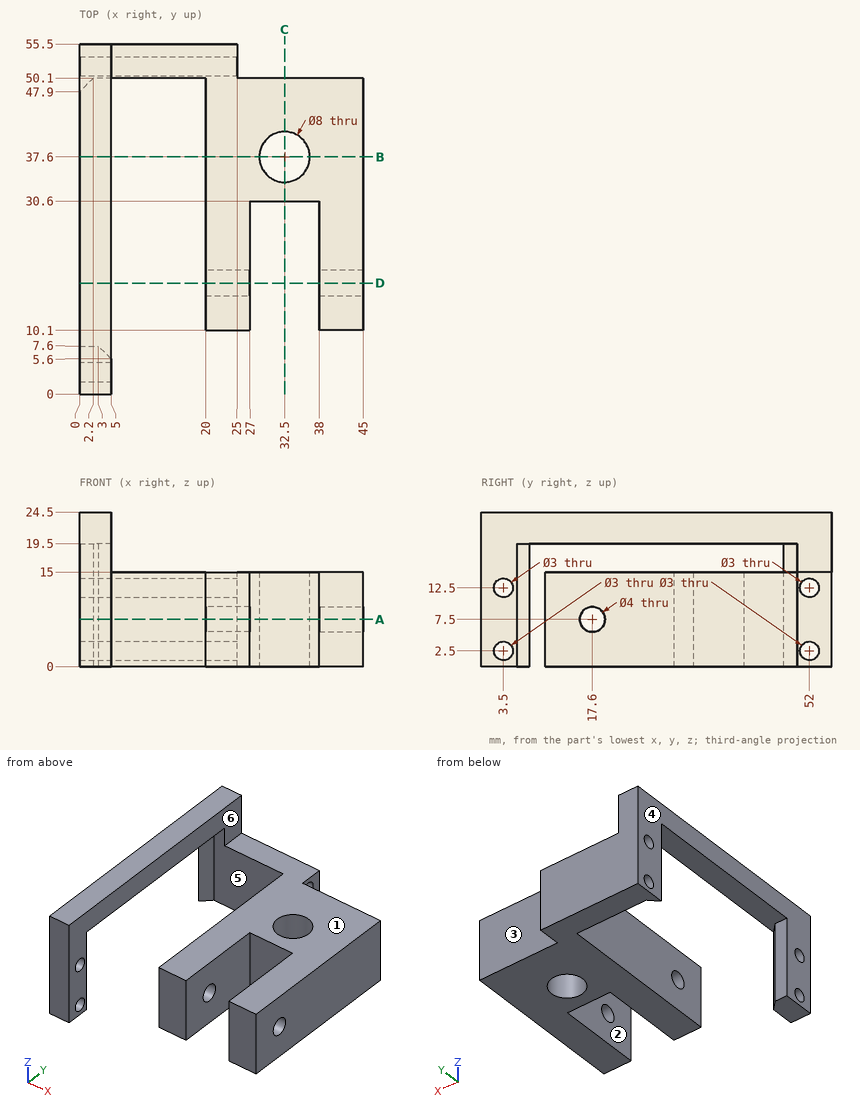
Could you check a few things on this drawing? It's one solid part, dimensions in mm from its lowest x, y, z. A direction names the side the tool comes from. Round coordinates to 2 decimals unless told otherwise and drop trailing zeros. Order: outer loops, then holes, each group sorted by start corner. A loop starts at its lowest first (then second) coordinate and runs counter-clockwise, first axis right, second up. Notation, with made-up numbers: M 32.25,88 L 74.25,88 A16 cw 74.25,113 Z; hole C -15.75,29.5 d5. An arc over 180 degrees is marked long. One line per question, with ' | ' between items. Start each with the question number.
(1) Suppose I cut it at C-C on x = 32.5. List the corners of the cut face in (y, z) for me, then the cut area to 4 significant figures.
(2) Suppose I cut it at B-B on y = 37.6. List the corners of the cut face in (x, z) for me, then the cut area to 3 significant figures.
(3) Thinking about a two-plate mould opening in X: for the marked faces 4, 5 and 6, which applies, +X half, -X half, draft (parallel to the pull), parting line (faces both ways), or undercut?
(4) Suppose I cut it at D-D on y = 17.6. List the corners of the cut face in (x, z) for me.
(5) Please list where these lines run through material, in increasing order: line 1 along Z through (x, y) = (7.25, 52); line 2 along Z through (x, y) = (38, 38.5); line 3 along Y through (x, z) = (32.5, 10.5).
(6) For P1, Ø12, axis at x = 33, z = 11, coming from the +Y side; P2, Ø2, axis at y = 39.5, z = 8.5, coming from the -X side; P3, Ø20, axis at x = 19, y = 32.5, coming from the +Z side; P4, Ø3.5, axis at y = 52, z = 2.5, coming from the -X side, each with a flat end and sliding along its axis, tell me the tip position at first contact or that it passes through.
(7) For the marked faces 1, 2 and 3, which set-ups out of +Z, -Z, +X, -X, +Y, -Y let a thin tool reach every point of the face, with its end or its side?
(8) Suppose I cut it at A-A on z = 7.5. List the corners of the cut face in (x, y) for me, then the cut area to 3 significant figures.
Geometry results:
1) outline: M 30.6,0 L 33.6,0 L 33.6,15 L 30.6,15 Z; M 41.6,0 L 50.1,0 L 50.1,15 L 41.6,15 Z | area: 172.5 mm²
2) outline: M 0,19.5 L 5,19.5 L 5,24.5 L 0,24.5 Z; M 20,0 L 28.5,0 L 28.5,15 L 20,15 Z; M 36.5,0 L 45,0 L 45,15 L 36.5,15 Z | area: 280 mm²
3) face 4: -X half | face 5: undercut | face 6: +X half
4) outline: M 0,19.5 L 5,19.5 L 5,24.5 L 0,24.5 Z; M 20,0 L 27,0 L 27,5.5 L 20,5.5 Z; M 20,9.5 L 27,9.5 L 27,15 L 20,15 Z; M 38,0 L 45,0 L 45,5.5 L 38,5.5 Z; M 38,9.5 L 45,9.5 L 45,15 L 38,15 Z
5) line 1: 0 to 1, 4 to 11, 14 to 15 | line 2: 0 to 15 | line 3: 30.6 to 33.6, 41.6 to 50.1
6) P1: y = 50.1 | P2: x = 20 | P3: z = 15 | P4: x = 0
7) face 1: +Z, +X, +Y, -Y | face 2: +Z, -Z, -Y | face 3: +Z, -Z, +X, +Y
8) outline: M 0,0 L 5,0 L 5,5.6 L 3,7.6 L 0,7.6 Z; M 0,47.9 L 2.2,50.1 L 20,50.1 L 20,19.6 L 27,19.6 L 27,30.6 L 38,30.6 L 38,19.6 L 45,19.6 L 45,50.1 L 25,50.1 L 25,55.5 L 0,55.5 Z; M 20,10.1 L 27,10.1 L 27,15.6 L 20,15.6 Z; M 38,10.1 L 45,10.1 L 45,15.6 L 38,15.6 Z; hole C 32.5,37.6 d8 | area: 842 mm²
